Geometry check sheet. Reference: the model listing, model coordinates, mm. A direction names the side the tool comes from. Give positions to 0.01 mm unless a question says otherwise; leave off trailing zeros. Loops run counter-clockwise (first coordinate to the right, second up) from the corner with the lowest first, then second, coordinate; pieces in that order, holes last. Notation, with made-up numbers: (34.5, -3.75) - (85.5, -3.75) arc R9 cw to (85.5, 0.25) - close; hole circle Ø1 at (-16, 9). An arc over 180 degrees is marked (long way). Write item = value, one per line. Start each with the question number.
from build123d import *

# Parameters (mm, degrees)
BOSS_EXTRUDE1_DEPTH      = 4.5
BOSS_EXTRUDE1_DEPTH_BACK = 4.5
SKETCH1_R                = 12
SKETCH3_RX               = 6
SKETCH3_RY               = 3.5
CUT_EXTRUDE1_REACH       = 98.896


with BuildPart() as part:
    # Sketch1 → Boss-Extrude1 (new, two sides: drawn at the far end of the back side and taken through both)
    with BuildSketch(Plane(origin=(0, 0, 0), x_dir=(0, 1, 0), z_dir=(0, 0, 1)).offset(-BOSS_EXTRUDE1_DEPTH_BACK)):
        with Locations(Location((0, 0, 0), (0, 0, 270))):
            Circle(SKETCH1_R)
    extrude(amount=BOSS_EXTRUDE1_DEPTH + BOSS_EXTRUDE1_DEPTH_BACK)

    # Sweep1: sweep along a path in Sketch2
    with BuildLine(Plane.YZ) as sweep1_path:
        Line((0, 0), (-20, 0))
        Line((-20, 0), (-31.5, 19.918584287))
        Line((-31.5, 19.918584287), (-86.5, 19.918584287))
    # Sketch3 → Sweep1 (sweep)
    with BuildSketch(Plane(origin=(0, 0, 0), x_dir=(-1, 0, 0), z_dir=(0, 1, 0))):
        with Locations((0, 0)):
            Ellipse(SKETCH3_RX, SKETCH3_RY)
    sweep(path=sweep1_path.line, transition=Transition.RIGHT)

    # Sketch4 → Revolve1 (revolve)
    with BuildSketch(Plane.XZ.offset(86.5)):
        with BuildLine():
            Line((0, 26.918584287), (0, 12.918584287))
            ThreePointArc((0, 12.918584287), (7, 19.918584287), (0, 26.918584287))
        make_face()
    revolve(axis=Axis((0, -86.5, 26.918584287), (0, 0, -1)))

    # Sketch5 → Cut-Extrude1 (cut, up to next)
    with BuildSketch(Plane.XY.offset(4.5), mode=Mode.PRIVATE) as cut_extrude1_sk1:
        Polygon((0, 6.363961031), (-6.363961031, 0), (0, -6.363961031), (6.363961031, 0), align=None)
    cut_extrude1_tool1 = extrude(cut_extrude1_sk1.sketch, amount=-CUT_EXTRUDE1_REACH, mode=Mode.PRIVATE) & part.part
    add(cut_extrude1_tool1.solids().sort_by_distance((0, 0, 4.5))[0], mode=Mode.SUBTRACT)


solid = part.part
1) Release check for a two-part mould opening along Y. For faces 1 (the face through (3.137, -3.227, 0.063)), 2 (the face through (5, -2, -4.5)) record: pulls with the +Y half, pulls with the -Y half, needs draft (parallel to the pull), parting line crosses it, or undercut.
2) Gauge pin test, flat ends, axial feed: P1, Ø3, axis at x = -6, y = -64.5, coming from the -Z side; P2, Ø5, axis at y = -70, z = 18, coming from the -X side; P3, Ø6, axis at x = -1, z = 20.5, coming from the -Y side; P4, Ø8, axis at x = 6.5, y = -24, coming from the -Z side. Record the tip position at first contact, or that the pin passes through.
3) Cross-section at A-A on y = -85. Enter the section's corners in (x, z).
4) Material ranges on line 1 along Z through (x, y) = (3.25, -7); line 2 along Y through (x, z) = (-2.25, 15.5); line 3 along Y through (x, z) = (-5.75, 0), recorded low to high.
5) Tool access check on faces 3 (the face through (5, -2, 4.5)), 4 (the face through (3.227, 3.137, 0.063)). Record the directions out of +Z, -Z, +X, -X, +Y, -Y that give a thin tool (end or side, any length) a straight path to the whole face; none if there is none.
Checked values:
q1.face_1 = undercut
q1.face_2 = needs draft
q2.P1 = 17.6
q2.P2 = -6
q2.P3 = -93.5
q2.P4 = -2.95
q3.outline = circle Ø13.67 at (0, 19.92)
q4.line_1 = -4.5 to 4.5
q4.line_2 = -91.44 to -81.56, -32.7 to -25.2
q4.line_3 = -21.15 to -0.61, 0.61 to 10.53
q5.face_3 = +Z, +X, -X, +Y
q5.face_4 = +Z, -Z
